For this review, take the finished solid that the model builds, in its own axes (mm). Face numbers are marked on the shaded views. A direction names the side the tool comes from. Coordinates: 2 decimals unless noted, no trailing zeros. Order: outer loops, then holes, each group sorted by start corner. A loop starts at its lowest first (then second) coordinate and runs counter-clockwise, first axis right, second up. Notation, with made-up numbers: M -26,85 L 15,85 A16 cw 15,105 Z; hole C 56,-38 d9. An arc over 180 degrees is marked long. Use CSV: the item, a comma, the result in double quotes.
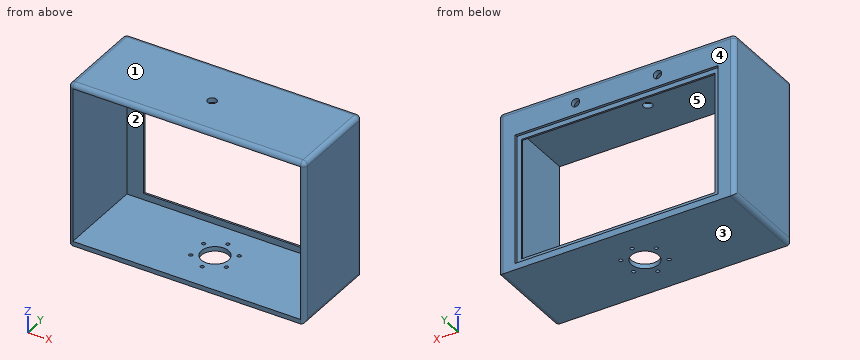
```python
from build123d import *

# Parameters (mm, degrees)
F0_W      = 260
F0_H      = 100
F1_DEPTH  = 180
F2_T      = -5
F3_W      = 223
F3_H      = 143
F3_W_2    = 212.9999995232
F3_H_2    = 132.9999995232
F4_DEPTH  = 3
F5_DEPTH  = 25
F3_R      = 4.5
F6_DEPTH  = 25
F7_R      = 2
F7_R_2    = 15
F8_DEPTH  = 25
F9_R      = 4.99999
F10_R     = 5
F11_DEPTH = 25


# Not quite as in the source:
# - a fillet or chamfer is up to 0.001 mm smaller than in the source, because OpenCascade refuses the exact size


with BuildPart() as f1:
    # F0 (on Top) → F1 (new body)
    with BuildSketch(Plane.XY):
        Rectangle(F0_W, F0_H)
    extrude(amount=F1_DEPTH)

    # F2
    f2_openings = [f1.faces().sort_by_distance(p)[0] for p in [
        (0, -50, 90),
    ]]
    offset(amount=F2_T, openings=f2_openings)

    # F3 (on face) → F4 (cut)
    with BuildSketch(Plane(origin=(0, 50, 0), x_dir=(-1, 0, 0), z_dir=(0, 1, 0))):
        with Locations((0, 78.5)):
            Rectangle(F3_W, F3_H)
        with Locations((0, 78.5)):
            Rectangle(F3_W_2, F3_H_2, mode=Mode.SUBTRACT)
    extrude(amount=-F4_DEPTH, mode=Mode.SUBTRACT)

    # F5 (cut): a face of the model
    f5_faces = [f1.faces().sort_by_distance(p)[0] for p in [
        (0, 50, 78.5),
    ]]
    extrude(f5_faces, amount=-F5_DEPTH, mode=Mode.SUBTRACT)

    # F3 (on face) → F6 (cut)
    with BuildSketch(Plane(origin=(0, 50, 0), x_dir=(-1, 0, 0), z_dir=(0, 1, 0))):
        with Locations((-45, 163)):
            Circle(F3_R)
        with Locations((45, 163)):
            Circle(F3_R)
    extrude(amount=-F6_DEPTH, mode=Mode.SUBTRACT)

    # F7 (on face) → F8 (cut)
    with BuildSketch(Plane(origin=(0, 0, 0), x_dir=(1, 0, 0), z_dir=(0, 0, -1))):
        with Locations((-19.5557196429, 11.2905)):
            Circle(F7_R)
        with Locations((0, 22.581)):
            Circle(F7_R)
        with Locations((19.5557196429, 11.2905)):
            Circle(F7_R)
        with Locations((19.5557196429, -11.2905)):
            Circle(F7_R)
        with Locations((0, -22.581)):
            Circle(F7_R)
        with Locations((-19.5557196429, -11.2905)):
            Circle(F7_R)
        Circle(F7_R_2)
    extrude(amount=-F8_DEPTH, mode=Mode.SUBTRACT)

    # F9 (radius 5 in the source; OpenCascade refuses exactly that, so slightly less here)
    f9_edges = [f1.edges().sort_by_distance(p)[0] for p in [
        (0, 50, 180),
        (-130, 0, 180),
        (-130, 50, 90),
        (-130, -50, 90),
        (-130, 0, 0),
        (0, -50, 180),
        (130, 0, 180),
        (130, -50, 90),
        (130, 50, 90),
        (130, 0, 0),
    ]]
    fillet(f9_edges, radius=F9_R)

    # F10 (on face) → F11 (cut)
    with BuildSketch(Plane.XY.offset(180)):
        with Locations((0, -5)):
            Circle(F10_R)
    extrude(amount=-F11_DEPTH, mode=Mode.SUBTRACT)


solid = f1.part
```
Item 1: Clearance check with flat-ended pins moving along their axes: pin 1 Ø3.5 at (y, z) = (48.5, 103) entering from +X; pin 2 Ø1.5 at (y, z) = (48, 62) entering from -X; pin 3 Ø3.5 at (x, y) = (-5, 48.5) entering from +Z. State where each tip first meets the part, or that it passes through.
Solutions:
pin 1,"x = 129.68"
pin 2,"x = -129.47"
pin 3,"z = 179.68"
Item 2: To check wall thickness, follow line 1 along Y through (x, z) = (0, 2.7); line 2 along X through (y, z) = (42.5, 90.5); line 3 along Z through (x, y) = (-23, 6). State the ranges of each line that lie inside material, in increasing order. Write a range as [from, to].
Solutions:
line 1,"[-50, -24.58], [-20.58, -15], [15, 20.58], [24.58, 50]"
line 2,"[-130, -125], [125, 130]"
line 3,"[0, 5], [175, 180]"
Item 3: For the marked faces 1 and 2, list the 3-axis set-ups (+Z, -Z, +X, -X, +Y, -Y) from which the entire face can be reached by the end or side of a thin tool; tool diameter is ignored.
Solutions:
face 1,"+Z, +X, -X, +Y, -Y"
face 2,"-Y"
Item 4: Draft analysis for pull direction Z (two halves, no side actions). For the marked faces 3, 4 and 5, state which applies: released by +Z, released by -Z, zero draft, split by the parting line, or undercut.
Solutions:
face 3,"released by -Z"
face 4,"zero draft"
face 5,"undercut"
Item 5: Add section C-C on y = 32. State the section outline as (x, z) points.
Solutions:
outline,"M -130,5 A5 ccw -125,0 L 125,0 A5 ccw 130,5 L 130,175 A5 ccw 125,180 L -125,180 A5 ccw -130,175 Z; hole M -125,5 L 125,5 L 125,175 L -125,175 Z"
Item 6: Add section A-A on x = 45. State how many separate pieces and enclosed holes the cut face has, and give its area (3 significant figures).
Solutions:
separate pieces,"3"
enclosed holes,"0"
area,"1,100 mm^2"
